from build123d import *

# Parameters (mm, degrees)
SKETCH2_R     = 1.25
SHAFT_DEPTH   = 15
PHILIPS_DEPTH = 1


with BuildPart() as part:
    # Sketch2 → Shaft (new body)
    with BuildSketch(Plane(origin=(0, 0, 0), x_dir=(1, 0, 0), z_dir=(0, 1, 0))):
        with Locations(Location((0, 0, 0), (0, 0, 270))):
            Circle(SKETCH2_R)
    extrude(amount=-SHAFT_DEPTH)

    # Sketch3 → Head (revolve)
    with BuildSketch(Plane.XY, mode=Mode.PRIVATE) as head_sk:
        with BuildLine():
            Line((0, 0), (0, 2.2))
            Line((0, 2.2), (1.65, 2.2))
            ThreePointArc((1.65, 2.2), (2.003553391, 2.053553391), (2.15, 1.7))
            Line((2.15, 1.7), (2.15, 0))
            Line((2.15, 0), (0, 0))
        make_face()
    revolve(head_sk.sketch.rotate(Axis((0, 0, 0), (0, 1, 0)), 90), axis=Axis((0, 0, 0), (0, 1, 0)))

    # Sketch5 → Philips (cut)
    with BuildSketch(Plane(origin=(0, 2.2, 0), x_dir=(1, 0, 0), z_dir=(0, 1, 0))):
        Polygon((-0.3, -1.15), (0.3, -1.15), (0.3, -0.3), (1.15, -0.3), (1.15, 0.3), (0.3, 0.3), (0.3, 1.15), (-0.3, 1.15), (-0.3, 0.3), (-1.15, 0.3), (-1.15, -0.3), (-0.3, -0.3), align=None)
    extrude(amount=-PHILIPS_DEPTH, mode=Mode.SUBTRACT)


solid = part.part
Design review of the part built by this model. Coordinates are the model's own, in mm. A direction names the side the tool comes from. Round coordinates to 2 decimals unless told otherwise and drop trailing zeros. Write each loop counter-clockwise with the first axis right and the second up, starting at its lowest first coordinate (ties: lowest second). Pieces come first, ordered by that corner, then holes.
Item 1: For pin 1 Ø0.7 at (y, z) = (2, 1) entering from -X; pin 2 Ø0.5 at (x, y) = (0, 2) entering from -Z; pin 3 Ø0.7 at (x, y) = (0.5, 1.5) entering from +Z; pin 4 Ø1.8 at (x, z) = (0.5, 0) entering from +Y, all flat-tipped, find the tip position at first contact; note any pin that passes through.
Item 2: For faces 1 (the flat face through (1, 0, -1)), 2 (the flat face through (0.7, 1.7, 0.3)), list the 3-axis set-ups (+Z, -Z, +X, -X, +Y, -Y) from which the entire face can be reached by the end or side of a thin tool; tool diameter is ignored.
Item 3: Consider section D-D on y = 1. Give the boundary of the cut face in (x, z).
Item 4: Consider section A-A on x = 0. Give the boundary of the cut face in (y, z), and give its area (3 significant figures).
Item 5: Draft analysis for pull direction Z (two halves, no side actions). For faces 3 (the flat face through (0, -15, 0)), 4 (the flat face through (-0.7, 1.7, -0.3)), 5 (the cylindrical face through (-0.09, 0.84, 2.15)), state which applies: released by +Z, released by -Z, zero draft, split by the parting line, or undercut.
Item 6: Wall thickness on L1, parallel to Z at x = 0.1, y = 1.5; L2, parallel to Z at x = -0.1, y = -8; L3, parallel to Y at x = 0.7, z = -1.4: over which ranges is each line inside the solid? List them lowest first.
Item 7: Consider section B-B on z = 0. Give the boundary of the cut face in (x, y), and give its area (3 significant figures).
Item 8: Consider section C-C on y = -9. Give the boundary of the cut face in (x, z), and give its area (3 significant figures).
Check values:
1. pin 1: stops at x = -2.02
1. pin 2: stops at z = -2.15
1. pin 3: stops at z = 2.14
1. pin 4: stops at y = 2.2
2. face 1: -Y
2. face 2: +Y
3. outline: circle Ø4.3 at (0, 0)
4. outline: (-15, -1.25) - (0, -1.25) - (0, -2.15) - (1.7, -2.15) arc R0.5 ccw to (2.2, -1.65) - (2.2, -1.15) - (1.2, -1.15) - (1.2, 1.15) - (2.2, 1.15) - (2.2, 1.65) arc R0.5 ccw to (1.7, 2.15) - (0, 2.15) - (0, 1.25) - (-15, 1.25) - close
4. area: 44.6 mm2
5. face 3: zero draft
5. face 4: undercut
5. face 5: split by the parting line
6. L1: z = -2.15 to -1.15, 1.15 to 2.15
6. L2: z = -1.25 to 1.25
6. L3: y = 0 to 2.2
7. outline: (-2.15, 0) - (-1.25, 0) - (-1.25, -15) - (1.25, -15) - (1.25, 0) - (2.15, 0) - (2.15, 1.7) arc R0.5 ccw to (1.65, 2.2) - (1.15, 2.2) - (1.15, 1.2) - (-1.15, 1.2) - (-1.15, 2.2) - (-1.65, 2.2) arc R0.5 ccw to (-2.15, 1.7) - close
7. area: 44.6 mm2
8. outline: circle Ø2.5 at (0, 0)
8. area: 4.91 mm2
